CAD build for the part. Positions are in the model's coordinates, mm. A direction names the side the tool comes from. Give positions to 0.01 mm unless a question says otherwise; leave off trailing zeros. Loops run counter-clockwise (first coordinate to the right, second up) from the corner with the lowest first, then second, coordinate; pieces in that order, holes last.
Item 1: Mould opens along Z. For faces 4 (the flat face through (-64, -1, -19.05)), 5 (the flat face through (-2, -1, -107.244)), 6 (the flat face through (-21, -1, -40.272)), 7 (the flat face through (-11.2, -1, -55)) say: released by +Z, released by -Z, zero draft, split by the parting line, or undercut.
Item 2: Which spindle directions (+Z, -Z, +X, -X, +Y, -Y) get a long thin tool onto all of the face, cutting with end or side? Do faces 1 (the flat face through (-11.2, -1, -75)), 2 (the flat face through (-3.1, -1, -75)), 3 (the flat face through (-89.122, -1, -21)). Say none if no direction does.
Item 3: Drop flat-ended pins along their axis: P1, Ø0.9, axis at x = -20.5, y = -1, coming from the +Z side; P2, Ø1.5, axis at x = -9, y = -1.5, coming from the -Z side; P3, Ø0.9, axis at y = -1, z = -73, coming from the +X side. Give the stop position or say it passes through.
Item 4: Saw through at B-B on x = -20.5. Give the cut face in (y, z), plus the area to 3 significant figures.
Item 5: Probe probe 1 along X at (y, z) = (-1.85, -99.5); probe 2 along X at (y, z) = (-1.4, -11.5); probe 3 along Z at (x, y) = (-58.5, -1.25). List the from-to ranges inside material, lowest first.
Item 6: Saw through at C-C on x = -74.5. Give the cut face in (y, z).
Item 7: Saw through at D-D on y = -1.9. Give the number of separate pieces and of enclosed holes in the cut face, plus the area to 3 significant figures.
Item 8: Saw through at A-A on z = -77.5. Give the cut face in (x, y).
from build123d import *

# Parameters (mm, degrees)
BOSS_EXTRUDE1_DEPTH = 3
SKETCH2_R           = 1.5875
CUT_EXTRUDE1_DEPTH  = 4
SKETCH4_W           = 10.2
SKETCH4_H           = 3.2
SKETCH4_W_2         = 3.2
SKETCH4_H_2         = 10.2
SKETCH4_W_3         = 12.25
CUT_EXTRUDE2_DEPTH  = 4


with BuildPart() as part:
    # Sketch1 → Boss-Extrude1 (new body)
    with BuildSketch(Plane(origin=(0, 0, 0), x_dir=(1, 0, 0), z_dir=(0, 1, 0))):
        Polygon((-129.394434203, 8.1), (-117.394434203, 8.1), (-117.394434203, 19.05), (-31.05, 19.05), (-31.05, 8.1), (-22.05, 8.1), (-22.05, 0), (0, 0), (0, 110.344434203), (-129.394434203, 110.344434203), align=None)
    extrude(amount=-BOSS_EXTRUDE1_DEPTH)

    # Sketch2 → Cut-Extrude1 (cut, through all)
    with BuildSketch(Plane(origin=(0, 0, 0), x_dir=(1, 0, 0), z_dir=(0, 1, 0))):
        with Locations((-58.354434203, 97.724434203)):
            Circle(SKETCH2_R)
        with Locations((-58.354434203, 69.784434203)):
            Circle(SKETCH2_R)
        with Locations((-110.424434203, 102.804434203)):
            Circle(SKETCH2_R)
        with Locations((-109.154434203, 54.544434203)):
            Circle(SKETCH2_R)
    extrude(amount=-CUT_EXTRUDE1_DEPTH, mode=Mode.SUBTRACT)

    # Sketch4 → Cut-Extrude2 (cut, through all)
    with BuildSketch(Plane(origin=(0, 0, 0), x_dir=(1, 0, 0), z_dir=(0, 1, 0))):
        Polygon((-126.294434203, 22.15), (-129.494434203, 22.15), (-129.494434203, 8), (-117.294434203, 8), (-117.294434203, 11.2), (-121.494434203, 11.2), (-121.494434203, 8.7), (-126.294434203, 8.7), align=None)
        with Locations((-74.222217102, 20.55)):
            Rectangle(SKETCH4_W, SKETCH4_H)
        with Locations((-94.222217102, 20.55)):
            Rectangle(SKETCH4_W, SKETCH4_H)
        with Locations((-54.222217102, 20.55)):
            Rectangle(SKETCH4_W, SKETCH4_H)
        Polygon((-26.95, 8.7), (-22.05, 8.7), (-22.05, 8), (-31.15, 8), (-31.15, 11.2), (-26.95, 11.2), align=None)
        with Locations((-9.6, 35.172217102)):
            Rectangle(SKETCH4_W_2, SKETCH4_H_2)
        with Locations((-16.025, 1.5)):
            Rectangle(SKETCH4_W_3, SKETCH4_H)
        with Locations((-9.6, 15.172217102)):
            Rectangle(SKETCH4_W_2, SKETCH4_H_2)
        with Locations((-1.5, 15.172217102)):
            Rectangle(SKETCH4_W_2, SKETCH4_H_2)
        with Locations((-1.5, 35.172217102)):
            Rectangle(SKETCH4_W_2, SKETCH4_H_2)
        with Locations((-20.55, 35.172217102)):
            Rectangle(SKETCH4_W_2, SKETCH4_H_2)
        with Locations((-1.5, 55.172217102)):
            Rectangle(SKETCH4_W_2, SKETCH4_H_2)
        with Locations((-20.55, 55.172217102)):
            Rectangle(SKETCH4_W_2, SKETCH4_H_2)
        with Locations((-1.5, 75.172217102)):
            Rectangle(SKETCH4_W_2, SKETCH4_H_2)
        with Locations((-20.55, 75.172217102)):
            Rectangle(SKETCH4_W_2, SKETCH4_H_2)
        with Locations((-1.5, 95.172217102)):
            Rectangle(SKETCH4_W_2, SKETCH4_H_2)
        with Locations((-20.55, 95.172217102)):
            Rectangle(SKETCH4_W_2, SKETCH4_H_2)
        with Locations((-9.6, 108.844434203)):
            Rectangle(SKETCH4_W_2, SKETCH4_H)
        with Locations((-1.5, 108.844434203)):
            Rectangle(SKETCH4_W_2, SKETCH4_H)
        with Locations((-9.6, 95.172217102)):
            Rectangle(SKETCH4_W_2, SKETCH4_H_2)
        with Locations((-9.6, 75.172217102)):
            Rectangle(SKETCH4_W_2, SKETCH4_H_2)
        with Locations((-9.6, 55.172217102)):
            Rectangle(SKETCH4_W_2, SKETCH4_H_2)
    extrude(amount=-CUT_EXTRUDE2_DEPTH, mode=Mode.SUBTRACT)


solid = part.part
Results below:
1. face 4: released by +Z
1. face 5: released by -Z
1. face 6: undercut
1. face 7: undercut
2. face 1: +Y, -Y
2. face 2: +X, +Y, -Y
2. face 3: +Z, +Y, -Y
3. P1: stops at z = -3.1
3. P2: stops at z = -107.24
3. P3: stops at x = -3.1
4. outline: (-3, -110.34) - (0, -110.34) - (0, -100.27) - (-3, -100.27) - close; (-3, -90.07) - (0, -90.07) - (0, -80.27) - (-3, -80.27) - close; (-3, -70.07) - (0, -70.07) - (0, -60.27) - (-3, -60.27) - close; (-3, -50.07) - (0, -50.07) - (0, -40.27) - (-3, -40.27) - close; (-3, -30.07) - (0, -30.07) - (0, -3.1) - (-3, -3.1) - close
4. area: 199 mm2
5. probe 1: x = -129.39 to -22.15, -18.95 to -11.2, -8 to -3.1
5. probe 2: x = -126.29 to -117.39, -31.05 to -11.2, -8 to -3.1
5. probe 3: z = -110.34 to -99.31, -96.14 to -71.37, -68.2 to -22.15
6. outline: (-3, -110.34) - (0, -110.34) - (0, -22.15) - (-3, -22.15) - close
7. separate pieces: 1
7. enclosed holes: 13
7. area: 11,800 mm2
8. outline: (-129.39, -3) - (-22.15, -3) - (-22.15, 0) - (-129.39, 0) - close; (-18.95, -3) - (-11.2, -3) - (-11.2, 0) - (-18.95, 0) - close; (-8, -3) - (-3.1, -3) - (-3.1, 0) - (-8, 0) - close
